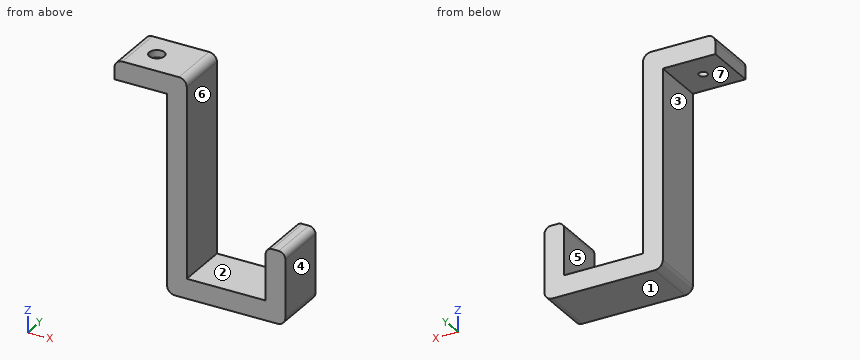
Autodesk Fusion 360 part; units mm, degrees
sketch "side" plane through (0, 0, 0) normal (0, 1, 0) x (1, 0, 0)
  line L0 (0, 0) -> (27.5, 0)
  line L1 (0, 0) -> (0, 7.5)
  line L2 (0, 7.5) -> (20, 7.5)
  line L3 (20, 7.5) -> (20, 82.5)
  line L4 (34.8526, 82.5) -> (20, 82.5)
  line L5 (34.8526, 82.5) -> (65, 82.5)
  line L6 (65, 82.5) -> (65, 55)
  line L7 (65, 55) -> (57.5, 55)
  line L8 (57.5, 55) -> (57.5, 75)
  line L9 (57.5, 75) -> (27.5, 75)
  line L10 (27.5, 75) -> (27.5, 0)
  dimension "d1" = 7.5
  dimension "d2" = 7.5
  dimension "d3" = 7.5
  dimension "d4" = 20
  dimension "d5" = 7.5
  dimension "d6" = 30
  dimension "d7" = 20
  dimension "d8" = 75
extrude "Extrude1" add sketch "side" along normal blind 20
sketch "top" plane through (0, 0, 0) normal (0, 0, 1) x (-1, 0, 0)
  line L0 (0, 0) -> (-27.5, 0)
  line L1 (-27.5, 0) -> (-27.5, -20)
  line L2 (-27.5, -20) -> (0, -20)
  line L3 (0, -20) -> (0, 0)
  line L4 (-13.75, -20) -> (-13.75, 0) construction
  circle A0 centre (-10.375, -10) radius 1.625
  circle A1 centre (-10.375, -10) radius 2.875
  line L5 (-10.375, -10) -> (0, -10) construction
  dimension "d11" = 3.25
  dimension "d12" = 5.75
  dimension "d27" = 7.5
fillet "Fillet1" radius 3 1 edges at (65, 10, -82.5)
fillet "Fillet2" radius 3 1 edges at (27.5, 10, 0)
fillet "Fillet3" radius 3 1 edges at (20, 10, -82.5)
fillet "Fillet4" radius 2.5 2 edges at (65, 10, -55) (57.5, 10, -55)
fillet "Fillet5" radius 3 1 edges at (0, 10, 0)
extrude "Extrude2" cut sketch "top" against normal up to surface (7.5 mm away) contours A0
extrude "Extrude3" cut sketch "top" against normal blind 2.75 contours A1
Read the model definition and answer for the solid it produces. Units are mm, in the model's axes. Face numbers are marked on the shaded views. A direction names the side the tool comes from. Round coordinates to 2 decimals unless told otherwise and drop trailing zeros. Write each loop counter-clockwise with the first axis right and the second up, starting at its lowest first coordinate (ties: lowest second). Pieces come first, ordered by that corner, then holes. Notation, with made-up numbers: (24.25, 89.25) - (71.25, 89.25) arc R11 cw to (71.25, 109.25) - close; hole circle Ø2 at (18, 75.25). An arc over 180 degrees is marked (long way). Use a Markdown table: item, result.
(1) The part is cut by section D-D (z = -45). Write down the section's boundary in (x, y).
Reported:
| item | result |
|---|---|
| outline | (20, 0) - (27.5, 0) - (27.5, 20) - (20, 20) - close |
(2) Each of these flat-tipped pins is pushed along its axis until it touches: pin 1 Ø6 at (y, z) = (12.5, -25.5) entering from -X; pin 2 Ø5 at (x, y) = (10.375, 10) entering from -Z; pin 3 Ø4 at (y, z) = (6, -51.5) entering from +X. Where does it stop, or does it pass through?
Reported:
| item | result |
|---|---|
| pin 1 | x = 20 |
| pin 2 | z = -7.5 |
| pin 3 | x = 27.5 |
(3) Straight lines are drawn through the part: line 1 along X through (y, z) = (10, -4.5); line 2 along Z through (x, y) = (4.5, 17); line 3 along Z through (x, y) = (29, 11.25). For each, find the intervals that lie inside material, in ascending order. Write a range as [from, to].
Reported:
| item | result |
|---|---|
| line 1 | [0, 8.75], [12, 27.5] |
| line 2 | [-7.5, 0] |
| line 3 | [-82.5, -75] |
(4) Which of the six approach directions +Z, -Z, +X, -X, +Y, -Y give full straight-line access (tool end or side, diameter ignored) to the marked faces 1, 2 and 3?
Reported:
| item | result |
|---|---|
| face 1 | -Z, +X, -X, +Y, -Y |
| face 2 | +Z, +Y, -Y |
| face 3 | -Z, -X, +Y, -Y |
(5) The mould has two halves that part along X. Classify the marked faces 4, 5, 6 and 7: released by +X, released by -X, zero draft, split by the parting line, or undercut.
Reported:
| item | result |
|---|---|
| face 4 | released by +X |
| face 5 | undercut |
| face 6 | undercut |
| face 7 | zero draft |
(6) The part is cut by section C-C (y = 13.75). Write down the section's boundary in (x, z), then the cut area to 3 significant figures.
Reported:
| item | result |
|---|---|
| outline | (0, -7.5) - (20, -7.5) - (20, -79.5) arc R3 ccw to (23, -82.5) - (62, -82.5) arc R3 ccw to (65, -79.5) - (65, -57.5) arc R2.5 ccw to (62.5, -55) - (60, -55) arc R2.5 ccw to (57.5, -57.5) - (57.5, -75) - (27.5, -75) - (27.5, -3) arc R3 ccw to (24.5, 0) - (3, 0) arc R3 ccw to (0, -3) - close |
| area | 1,190 mm2 |
(7) The part is cut by section B-B (y = 10). Write down the section's boundary in (x, z), then the cut area to 3 significant figures.
Reported:
| item | result |
|---|---|
| outline | (0, -7.5) - (8.75, -7.5) - (8.75, -2.75) - (7.5, -2.75) - (7.5, 0) - (3, 0) arc R3 ccw to (0, -3) - close; (12, -7.5) - (20, -7.5) - (20, -79.5) arc R3 ccw to (23, -82.5) - (62, -82.5) arc R3 ccw to (65, -79.5) - (65, -57.5) arc R2.5 ccw to (62.5, -55) - (60, -55) arc R2.5 ccw to (57.5, -57.5) - (57.5, -75) - (27.5, -75) - (27.5, -3) arc R3 ccw to (24.5, 0) - (13.25, 0) - (13.25, -2.75) - (12, -2.75) - close |
| area | 1,160 mm2 |
(8) The part is cut by section A-A (z = -72). Write down the section's boundary in (x, y).
Reported:
| item | result |
|---|---|
| outline | (20, 0) - (27.5, 0) - (27.5, 20) - (20, 20) - close; (57.5, 0) - (65, 0) - (65, 20) - (57.5, 20) - close |
